```python
from build123d import *

# Parameters (mm, degrees)
STOCK_2D1LAYER_1_START       = -45
STOCK_2D1LAYER_1_OUTLINE_W   = 200
STOCK_2D1LAYER_1_OUTLINE_H   = 4
STOCK_2D1LAYER_1_DEPTH       = 45
STOCK_2D1LAYER_1_START_2     = -135
STOCK_2D1LAYER_1_2_OUTLINE_W = 50
STOCK_2D1LAYER_1_2_OUTLINE_H = 4
STOCK_2D1LAYER_1_2_DEPTH     = 90
SKETCH1_W                    = 89
SKETCH1_H                    = 4
CUT_EXTRUDE1_DEPTH           = 1


# Read off the part's stored shape, not the designer's step: Stock-2D1Layer-1
with BuildPart() as part:
    # Stock-2D1Layer-1 outline → Stock-2D1Layer-1 (new body)
    with BuildSketch(Plane.XY.offset(STOCK_2D1LAYER_1_START)):
        with Locations((100, 6)):
            Rectangle(STOCK_2D1LAYER_1_OUTLINE_W, STOCK_2D1LAYER_1_OUTLINE_H)
    extrude(amount=STOCK_2D1LAYER_1_DEPTH)

    # Stock-2D1Layer-1 2 outline → Stock-2D1Layer-1 2 (add)
    with BuildSketch(Plane.XY.offset(STOCK_2D1LAYER_1_START_2)):
        with Locations((25, 6)):
            Rectangle(STOCK_2D1LAYER_1_2_OUTLINE_W, STOCK_2D1LAYER_1_2_OUTLINE_H)
    extrude(amount=STOCK_2D1LAYER_1_2_DEPTH)

    # Sketch1 → Cut-Extrude1 (cut)
    with BuildSketch(Plane(origin=(50, 0, 0), x_dir=(0, 0, -1), z_dir=(1, 0, 0))):
        with Locations((90.5, 6)):
            Rectangle(SKETCH1_W, SKETCH1_H)
    extrude(amount=-CUT_EXTRUDE1_DEPTH, mode=Mode.SUBTRACT)


solid = part.part
```
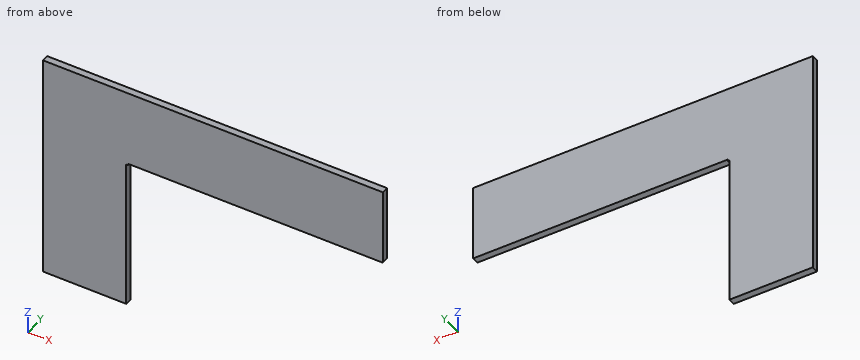
Input: part model. Units: mm. Frame: model coordinates. Give positions to 0.01 mm unless a question says otherwise; leave off trailing zeros. Loops run counter-clockwise (first coordinate to the right, second up) from the corner with the lowest first, then second, coordinate; pieces in that order, holes last. Notation, with made-up numbers: M 65,73 L 108,73 A5 ccw 108,79 Z; hole C -16.75,14.5 d10. An arc over 180 degrees is marked long. Answer as CSV lines item,"result". Start each with the question number.
1. Section C-C on z = -66. Return loops of the section in (x, y), plus the area to 3 significant figures.
2. Section B-B on x = 95. Return loops of the section in (y, z).
3. Pin query (flat end, axial travel): P1, Ø0.5, axis at y = 5.5, z = -45.5, coming from the +X side; P2, Ø0.8, axis at x = 49.5, y = 6.5, coming from the -Z side; P3, Ø2, axis at y = 5, z = -117.5, coming from the +X side. Return the tip coordinate at first contact, or that it passes through.
4. Section A-A on y = 7.1. Return loops of the section in (x, z).
5. Line query: L1, parallel to X at y = 7.85, z = -125; L2, parallel to Z at x = 173, y = 7.55. Output: solid intervals per line, ascending.
Computed values:
1,outline,"M 0,4 L 49,4 L 49,8 L 0,8 Z"
1,area,"196 mm²"
2,outline,"M 4,-45 L 8,-45 L 8,0 L 4,0 Z"
3,P1,"stops at x = 50"
3,P2,"stops at z = -46"
3,P3,"stops at x = 49"
4,outline,"M 0,-135 L 49,-135 L 49,-46 L 50,-46 L 50,-45 L 200,-45 L 200,0 L 0,0 Z"
5,L1,"x = 0 to 49"
5,L2,"z = -45 to 0"
